Check sheet for the modelled part. Datum: model origin and axes. Units: mm. A direction names the side the tool comes from. Give positions to 0.01 mm unless a question says otherwise; leave off trailing zeros. Order: outer loops, then holes, each group sorted by start corner. A loop starts at its lowest first (then second) coordinate and runs counter-clockwise, first axis right, second up.
Autodesk Inventor part; units mm, degrees
ref_plane "YZ Plane" through (0, 0, 0) normal (1, 0, 0) x (0, 1, 0)
ref_plane "XZ Plane" through (0, 0, 0) normal (0, 1, 0) x (-1, 0, 0)
ref_plane "XY Plane" through (0, 0, 0) normal (0, 0, 1) x (1, 0, 0)
sketch "Náčrt1" plane through (0, 0, 0) normal (0, 0, 1) x (1, 0, 0)
  line L0 (0, 0) -> (19.1477, 0)
  line L1 (0, 4) -> (0, 16.5)
  line L2 (0, 16.5) -> (8, 16.5)
  line L3 (8, 16.5) -> (8, 10.385)
  line L4 (8.4, 9.985) -> (54, 9.985)
  line L5 (54, 9.985) -> (54, 8.9)
  line L6 (54.4, 8.5) -> (82, 8.5)
  line L7 (82, 8.5) -> (82, 4)
  line L8 (82, 4) -> (0, 4)
  arc A0 (8, 10.385) -> (8.4, 9.985) centre (8.4, 10.385) ccw
  arc A1 (54, 8.9) -> (54.4, 8.5) centre (54.4, 8.9) ccw
  point P0 (54, 8.5)
  point P1 (8, 9.985)
  dimension "d0" = 33
  dimension "d1" = 82
  dimension "d2" = 28
  dimension "d5" = 17
  dimension "d6" = 8
  dimension "d7" = 19.97
  dimension "d8" = 74
  dimension "d39" = 8
  dimension "d40" = 46
  dimension "d41" = 0.4
  dimension "d42" = 0.4
revolve "Rotace1" add sketch "Náčrt1" angle 360 about axis through (0, 0, 0) along (1, 0, 0)
thread "Závit1"
chamfer "Zkosení1" distance 0.5 angle 45 1 edges at (0, -16.5, 0)
chamfer "Zkosení2" distance 0.5 angle 45 1 edges at (8, -16.5, 0)
chamfer "Zkosení3" distance 1 angle 30 1 edges at (0, -4, 0) measured on face at (54.6667, 3.987, -0.3219)
chamfer "Zkosení4" distance 1 angle 30 1 edges at (82, -4, 0) measured on face at (55, 3.987, -0.3219)
chamfer "Zkosení5" distance 0.5 angle 45 1 edges at (82, -8.5, 0)
sketch "Náčrt2" plane through (0, 0, 0) normal (-1, 0, 0) x (0, 0, 1)
  line L0 (-15, 6.8739) -> (-17.8524, 6.8739)
  line L1 (-17.8524, 6.8739) -> (-17.8524, -6.8739)
  line L2 (-17.8524, -6.8739) -> (-15, -6.8739)
  line L3 (-15, -6.8739) -> (-15, 6.8739)
  line L4 (19.6486, 6.8739) -> (15, 6.8739)
  line L5 (15, 6.8739) -> (15, -6.8739)
  line L6 (15, -6.8739) -> (19.6486, -6.8739)
  line L7 (19.6486, -6.8739) -> (19.6486, 6.8739)
  line L8 (0, 0) -> (0, -4.618) construction
  circle A0 centre (0, 0) radius 16.5 construction
  dimension "d29" = 30
extrude "Vysunutí1" cut sketch "Náčrt2" against normal through all
equation "\"Rozmer_A\" = d0"
equation "\"Rozmer_B\" = 0"
equation "\"Rozmer_C\" = 0"
equation "\"Rozmer_D\" = d1"
properties part number "NA-45-h-Crown-277" material "16 341"
1) Material ranges on L1, parallel to Z at x = 18.5, y = 0 (3 decimals); L2, parallel to Y at x = 13, z = 1; L3, parallel to X at y = 12.5, z = -4.5, recorded low to high.
Recorded:
L1: z = -9.985 to -4, 4 to 9.985
L2: y = -9.93 to -3.87, 3.87 to 9.93
L3: x = 0 to 8
2) Set-up check for faces 1 (the face through (54, -7, -6)), 2 (the face through (7.86, -16.14, -0.27)): record each of +Z, -Z, +X, -X, +Y, -Y from which the full face is reachable in a straight line by a thin tool's end or side.
Recorded:
face 1: +X
face 2: +X, -Y
3) Draft check along Z on faces 3 (the face through (40.44, -0.867, 3.905)), 4 (the face through (4.049, -16.498, 0.264)), 5 (the face through (4, 0, -15)). Enter one of: +Z half, -Z half, draft (parallel to the pull), parting line (faces both ways), or undercut.
Recorded:
face 3: undercut
face 4: parting line
face 5: -Z half
4) Section check C-C, the plane x = 25. Record the cut outline in (y, z) (3 decimals), then the cut area to 3 significant figures.
Recorded:
outline: circle Ø19.97 at (0, 0); hole circle Ø8 at (0, 0)
area: 263 mm2
5) Depth check by flat-ended pin: pin 1 Ø3 at (x, y) = (32.5, 7) entering from +Z; pin 2 Ø8 at (x, z) = (16.5, 9.5) entering from +Y; pin 3 Ø12 at (x, y) = (36, -13) entering from +Z. Enter the tip coordinate at first touch or a pass-through.
Recorded:
pin 1: stops at z = 8.33
pin 2: stops at y = 8.33
pin 3: stops at z = 7.12
6) Section check A-A, the plane y = 0. Record the cut outline in (x, z) (3 decimals), then the cut area to 3 significant figures.
Recorded:
outline: (0, -15) - (8, -15) - (8, -10.385) arc R0.4 cw to (8.4, -9.985) - (54, -9.985) - (54, -8.9) arc R0.4 cw to (54.4, -8.5) - (81.5, -8.5) - (82, -8) - (82, -4.577) - (81, -4) - (1, -4) - (0, -4.577) - close; (0, 4.577) - (1, 4) - (81, 4) - (82, 4.577) - (82, 8) - (81.5, 8.5) - (54.4, 8.5) arc R0.4 cw to (54, 8.9) - (54, 9.985) - (8.4, 9.985) arc R0.4 cw to (8, 10.385) - (8, 15) - (0, 15) - close
area: 977 mm2
